For this review, take the finished solid that the model builds, in its own axes (mm). Give positions to 0.01 mm unless a question says otherwise; leave off trailing zeros.
```python
from build123d import *

# Parameters (mm, degrees)
F0_W     = 101.6
F0_H     = 63.5
F1_DEPTH = 1.27


with BuildPart() as f1:
    # F0 (on Front) → F1 (new body)
    with BuildSketch(Plane.XZ):
        with Locations((-15.1200704277, 17.3774155871)):
            Rectangle(F0_W, F0_H)
        Polygon((-54.0476633337, 29.0188750451), (-54.0476633337, 27.9393295906), (-59.8362996974, 27.9393295906), (-59.8362996974, 38.3234204997), (-54.0476633337, 38.3234204997), (-54.0476633337, 37.2506932269), (-58.6294815156, 37.2506932269), (-58.6294815156, 33.9052386815), (-54.324936061, 33.9052386815), (-54.324936061, 32.8393295906), (-58.6294815156, 32.8393295906), (-58.6294815156, 29.0188750451), align=None, mode=Mode.SUBTRACT)
        with BuildLine():
            Line((-45.4181178792, 27.9393295906), (-46.5976633337, 27.9393295906))
            Line((-46.5976633337, 27.9393295906), (-46.5976633337, 32.9756932269))
            add(Edge.make_bspline(
                [(-46.5976633337, 32.9756932269), (-46.5976633337, 33.9256932269), (-47.0306178792, 34.3950114088)],
                knots=[0, 0, 0, 1, 1, 1], degree=2))
            add(Edge.make_bspline(
                [(-47.0306178792, 34.3950114088), (-47.4635724247, 34.8643295906), (-48.3885724247, 34.8643295906)],
                knots=[0, 0, 0, 1, 1, 1], degree=2))
            add(Edge.make_bspline(
                [(-48.3885724247, 34.8643295906), (-49.6090269701, 34.8643295906), (-50.1772087883, 34.2041023179)],
                knots=[0, 0, 0, 1, 1, 1], degree=2))
            add(Edge.make_bspline(
                [(-50.1772087883, 34.2041023179), (-50.7453906065, 33.5438750451), (-50.7453906065, 32.0234204997)],
                knots=[0, 0, 0, 1, 1, 1], degree=2))
            Line((-50.7453906065, 32.0234204997), (-50.7453906065, 27.9393295906))
            Line((-50.7453906065, 27.9393295906), (-51.924936061, 27.9393295906))
            Line((-51.924936061, 27.9393295906), (-51.924936061, 35.7234204997))
            Line((-51.924936061, 35.7234204997), (-50.9658451519, 35.7234204997))
            Line((-50.9658451519, 35.7234204997), (-50.774936061, 34.6575114088))
            Line((-50.774936061, 34.6575114088), (-50.7181178792, 34.6575114088))
            add(Edge.make_bspline(
                [(-50.7181178792, 34.6575114088), (-50.3544815156, 35.2325114088), (-49.7010724247, 35.5495568633)],
                knots=[0, 0, 0, 1, 1, 1], degree=2))
            add(Edge.make_bspline(
                [(-49.7010724247, 35.5495568633), (-49.0476633337, 35.8666023179), (-48.2453906065, 35.8666023179)],
                knots=[0, 0, 0, 1, 1, 1], degree=2))
            add(Edge.make_bspline(
                [(-48.2453906065, 35.8666023179), (-46.8385724247, 35.8666023179), (-46.1283451519, 35.1881932269)],
                knots=[0, 0, 0, 1, 1, 1], degree=2))
            add(Edge.make_bspline(
                [(-46.1283451519, 35.1881932269), (-45.4181178792, 34.509784136), (-45.4181178792, 33.0166023179)],
                knots=[0, 0, 0, 1, 1, 1], degree=2))
            Line((-45.4181178792, 33.0166023179), (-45.4181178792, 27.9393295906))
        make_face(mode=Mode.SUBTRACT)
        with BuildLine():
            Line((-37.3362996974, 27.9393295906), (-38.2112996974, 27.9393295906))
            Line((-38.2112996974, 27.9393295906), (-38.4453906065, 29.0484204997))
            Line((-38.4453906065, 29.0484204997), (-38.5022087883, 29.0484204997))
            add(Edge.make_bspline(
                [(-38.5022087883, 29.0484204997), (-39.0840269701, 28.3166023179), (-39.662436061, 28.0563750451)],
                knots=[0, 0, 0, 1, 1, 1], degree=2))
            add(Edge.make_bspline(
                [(-39.662436061, 28.0563750451), (-40.2408451519, 27.7961477724), (-41.1090269701, 27.7961477724)],
                knots=[0, 0, 0, 1, 1, 1], degree=2))
            add(Edge.make_bspline(
                [(-41.1090269701, 27.7961477724), (-42.2658451519, 27.7961477724), (-42.9226633337, 28.3938750451)],
                knots=[0, 0, 0, 1, 1, 1], degree=2))
            add(Edge.make_bspline(
                [(-42.9226633337, 28.3938750451), (-43.5794815156, 28.9916023179), (-43.5794815156, 30.0916023179)],
                knots=[0, 0, 0, 1, 1, 1], degree=2))
            add(Edge.make_bspline(
                [(-43.5794815156, 30.0916023179), (-43.5794815156, 32.4484204997), (-39.8090269701, 32.5620568633)],
                knots=[0, 0, 0, 1, 1, 1], degree=2))
            Line((-39.8090269701, 32.5620568633), (-38.4885724247, 32.6052386815))
            Line((-38.4885724247, 32.6052386815), (-38.4885724247, 33.0893295906))
            add(Edge.make_bspline(
                [(-38.4885724247, 33.0893295906), (-38.4885724247, 34.0052386815), (-38.8817542428, 34.4416023179)],
                knots=[0, 0, 0, 1, 1, 1], degree=2))
            add(Edge.make_bspline(
                [(-38.8817542428, 34.4416023179), (-39.274936061, 34.8779659542), (-40.1431178792, 34.8779659542)],
                knots=[0, 0, 0, 1, 1, 1], degree=2))
            add(Edge.make_bspline(
                [(-40.1431178792, 34.8779659542), (-41.1158451519, 34.8779659542), (-42.3431178792, 34.2825114088)],
                knots=[0, 0, 0, 1, 1, 1], degree=2))
            Line((-42.3431178792, 34.2825114088), (-42.7067542428, 35.184784136))
            add(Edge.make_bspline(
                [(-42.7067542428, 35.184784136), (-42.1317542428, 35.4961477724), (-41.4465269701, 35.6734204997)],
                knots=[0, 0, 0, 1, 1, 1], degree=2))
            add(Edge.make_bspline(
                [(-41.4465269701, 35.6734204997), (-40.7612996974, 35.8506932269), (-40.0703906065, 35.8506932269)],
                knots=[0, 0, 0, 1, 1, 1], degree=2))
            add(Edge.make_bspline(
                [(-40.0703906065, 35.8506932269), (-38.6794815156, 35.8506932269), (-38.0078906065, 35.2336477724)],
                knots=[0, 0, 0, 1, 1, 1], degree=2))
            add(Edge.make_bspline(
                [(-38.0078906065, 35.2336477724), (-37.3362996974, 34.6166023179), (-37.3362996974, 33.2529659542)],
                knots=[0, 0, 0, 1, 1, 1], degree=2))
            Line((-37.3362996974, 33.2529659542), (-37.3362996974, 27.9393295906))
        make_face(mode=Mode.SUBTRACT)
        with BuildLine():
            add(Edge.make_bspline(
                [(-29.6885724247, 28.9825114088), (-30.5044815156, 27.7961477724), (-32.1453906065, 27.7961477724)],
                knots=[0, 0, 0, 1, 1, 1], degree=2))
            add(Edge.make_bspline(
                [(-32.1453906065, 27.7961477724), (-33.6522087883, 27.7961477724), (-34.4976633337, 28.8552386815)],
                knots=[0, 0, 0, 1, 1, 1], degree=2))
            add(Edge.make_bspline(
                [(-34.4976633337, 28.8552386815), (-35.3431178792, 29.9143295906), (-35.3431178792, 31.809784136)],
                knots=[0, 0, 0, 1, 1, 1], degree=2))
            add(Edge.make_bspline(
                [(-35.3431178792, 31.809784136), (-35.3431178792, 33.7211477724), (-34.4908451519, 34.7938750451)],
                knots=[0, 0, 0, 1, 1, 1], degree=2))
            add(Edge.make_bspline(
                [(-34.4908451519, 34.7938750451), (-33.6385724247, 35.8666023179), (-32.1181178792, 35.8666023179)],
                knots=[0, 0, 0, 1, 1, 1], degree=2))
            add(Edge.make_bspline(
                [(-32.1181178792, 35.8666023179), (-30.5203906065, 35.8666023179), (-29.6612996974, 34.6575114088)],
                knots=[0, 0, 0, 1, 1, 1], degree=2))
            Line((-29.6612996974, 34.6575114088), (-29.5953906065, 34.6575114088))
            Line((-29.5953906065, 34.6575114088), (-29.424936061, 35.7234204997))
            Line((-29.424936061, 35.7234204997), (-28.4953906065, 35.7234204997))
            Line((-28.4953906065, 35.7234204997), (-28.4953906065, 24.4438750451))
            Line((-28.4953906065, 24.4438750451), (-29.674936061, 24.4438750451))
            Line((-29.674936061, 24.4438750451), (-29.674936061, 27.7756932269))
            add(Edge.make_bspline(
                [(-29.674936061, 27.7756932269), (-29.674936061, 28.4870568633), (-29.5953906065, 28.9825114088)],
                knots=[0, 0, 0, 1, 1, 1], degree=2))
            Line((-29.5953906065, 28.9825114088), (-29.6885724247, 28.9825114088))
        make_face(mode=Mode.SUBTRACT)
        with BuildLine():
            Line((-26.0794815156, 35.7234204997), (-24.8862996974, 35.7234204997))
            Line((-24.8862996974, 35.7234204997), (-24.8862996974, 30.6734204997))
            add(Edge.make_bspline(
                [(-24.8862996974, 30.6734204997), (-24.8862996974, 29.7211477724), (-24.4533451519, 29.2529659542)],
                knots=[0, 0, 0, 1, 1, 1], degree=2))
            add(Edge.make_bspline(
                [(-24.4533451519, 29.2529659542), (-24.0203906065, 28.784784136), (-23.0976633337, 28.784784136)],
                knots=[0, 0, 0, 1, 1, 1], degree=2))
            add(Edge.make_bspline(
                [(-23.0976633337, 28.784784136), (-21.874936061, 28.784784136), (-21.3112996974, 29.4518295906)],
                knots=[0, 0, 0, 1, 1, 1], degree=2))
            add(Edge.make_bspline(
                [(-21.3112996974, 29.4518295906), (-20.7476633337, 30.1188750451), (-20.7476633337, 31.6325114088)],
                knots=[0, 0, 0, 1, 1, 1], degree=2))
            Line((-20.7476633337, 31.6325114088), (-20.7476633337, 35.7234204997))
            Line((-20.7476633337, 35.7234204997), (-19.5681178792, 35.7234204997))
            Line((-19.5681178792, 35.7234204997), (-19.5681178792, 27.9393295906))
            Line((-19.5681178792, 27.9393295906), (-20.5408451519, 27.9393295906))
            Line((-20.5408451519, 27.9393295906), (-20.7112996974, 28.9825114088))
            Line((-20.7112996974, 28.9825114088), (-20.774936061, 28.9825114088))
            add(Edge.make_bspline(
                [(-20.774936061, 28.9825114088), (-21.1362996974, 28.4075114088), (-21.7794815156, 28.1018295906)],
                knots=[0, 0, 0, 1, 1, 1], degree=2))
            add(Edge.make_bspline(
                [(-21.7794815156, 28.1018295906), (-22.4226633337, 27.7961477724), (-23.2476633337, 27.7961477724)],
                knots=[0, 0, 0, 1, 1, 1], degree=2))
            add(Edge.make_bspline(
                [(-23.2476633337, 27.7961477724), (-24.6681178792, 27.7961477724), (-25.3737996974, 28.4711477724)],
                knots=[0, 0, 0, 1, 1, 1], degree=2))
            add(Edge.make_bspline(
                [(-25.3737996974, 28.4711477724), (-26.0794815156, 29.1461477724), (-26.0794815156, 30.6302386815)],
                knots=[0, 0, 0, 1, 1, 1], degree=2))
            Line((-26.0794815156, 30.6302386815), (-26.0794815156, 35.7234204997))
        make_face(mode=Mode.SUBTRACT)
        with BuildLine():
            Line((-11.4067542428, 27.9393295906), (-12.2817542428, 27.9393295906))
            Line((-12.2817542428, 27.9393295906), (-12.5158451519, 29.0484204997))
            Line((-12.5158451519, 29.0484204997), (-12.5726633337, 29.0484204997))
            add(Edge.make_bspline(
                [(-12.5726633337, 29.0484204997), (-13.1544815156, 28.3166023179), (-13.7328906065, 28.0563750451)],
                knots=[0, 0, 0, 1, 1, 1], degree=2))
            add(Edge.make_bspline(
                [(-13.7328906065, 28.0563750451), (-14.3112996974, 27.7961477724), (-15.1794815156, 27.7961477724)],
                knots=[0, 0, 0, 1, 1, 1], degree=2))
            add(Edge.make_bspline(
                [(-15.1794815156, 27.7961477724), (-16.3362996974, 27.7961477724), (-16.9931178792, 28.3938750451)],
                knots=[0, 0, 0, 1, 1, 1], degree=2))
            add(Edge.make_bspline(
                [(-16.9931178792, 28.3938750451), (-17.649936061, 28.9916023179), (-17.649936061, 30.0916023179)],
                knots=[0, 0, 0, 1, 1, 1], degree=2))
            add(Edge.make_bspline(
                [(-17.649936061, 30.0916023179), (-17.649936061, 32.4484204997), (-13.8794815156, 32.5620568633)],
                knots=[0, 0, 0, 1, 1, 1], degree=2))
            Line((-13.8794815156, 32.5620568633), (-12.5590269701, 32.6052386815))
            Line((-12.5590269701, 32.6052386815), (-12.5590269701, 33.0893295906))
            add(Edge.make_bspline(
                [(-12.5590269701, 33.0893295906), (-12.5590269701, 34.0052386815), (-12.9522087883, 34.4416023179)],
                knots=[0, 0, 0, 1, 1, 1], degree=2))
            add(Edge.make_bspline(
                [(-12.9522087883, 34.4416023179), (-13.3453906065, 34.8779659542), (-14.2135724247, 34.8779659542)],
                knots=[0, 0, 0, 1, 1, 1], degree=2))
            add(Edge.make_bspline(
                [(-14.2135724247, 34.8779659542), (-15.1862996974, 34.8779659542), (-16.4135724247, 34.2825114088)],
                knots=[0, 0, 0, 1, 1, 1], degree=2))
            Line((-16.4135724247, 34.2825114088), (-16.7772087883, 35.184784136))
            add(Edge.make_bspline(
                [(-16.7772087883, 35.184784136), (-16.2022087883, 35.4961477724), (-15.5169815156, 35.6734204997)],
                knots=[0, 0, 0, 1, 1, 1], degree=2))
            add(Edge.make_bspline(
                [(-15.5169815156, 35.6734204997), (-14.8317542428, 35.8506932269), (-14.1408451519, 35.8506932269)],
                knots=[0, 0, 0, 1, 1, 1], degree=2))
            add(Edge.make_bspline(
                [(-14.1408451519, 35.8506932269), (-12.749936061, 35.8506932269), (-12.0783451519, 35.2336477724)],
                knots=[0, 0, 0, 1, 1, 1], degree=2))
            add(Edge.make_bspline(
                [(-12.0783451519, 35.2336477724), (-11.4067542428, 34.6166023179), (-11.4067542428, 33.2529659542)],
                knots=[0, 0, 0, 1, 1, 1], degree=2))
            Line((-11.4067542428, 33.2529659542), (-11.4067542428, 27.9393295906))
        make_face(mode=Mode.SUBTRACT)
    extrude(amount=F1_DEPTH)


solid = f1.part
```
Item 1: For L1, parallel to X at y = -0.85, z = 36.5; L2, parallel to Z at x = -13.5, y = -1; L3, parallel to Z at x = -15, y = -0.65, list the stretches that pass through material, from the lowest coordinate up.
Answer:
L1: x = -65.92 to -59.84, -58.63 to 35.68
L2: z = -14.37 to 28.18, 32.57 to 34.78, 35.81 to 49.13
L3: z = -14.37 to 27.8, 32.47 to 34.79, 35.78 to 49.13
Item 2: Take a section at A-A on y = -0.65. State how many separate pieces and enclosed holes the cut face has, and give its area (3 significant figures).
Answer:
separate pieces: 1
enclosed holes: 6
area: 6,260 mm2
Item 3: Clearance check with a flat-ended pin moving along its axis: pin 1 Ø1 at (x, z) = (8.5, 24) entering from +Y. State where the tip first meets the part, or that it passes through.
Answer:
pin 1: stops at y = 0
